The figure shows three views and two pictorial views of one solid part (mm, origin at its lowest corner). Answer the questions. A direction names the side the tool comes from. Coordinates: 2 decimals unless noted, no trailing zeros. Order: outer loops, then holes, each group sorted by start corner. A loop starts at its lowest first (then second) coordinate and runs counter-clockwise, first axis right, second up.
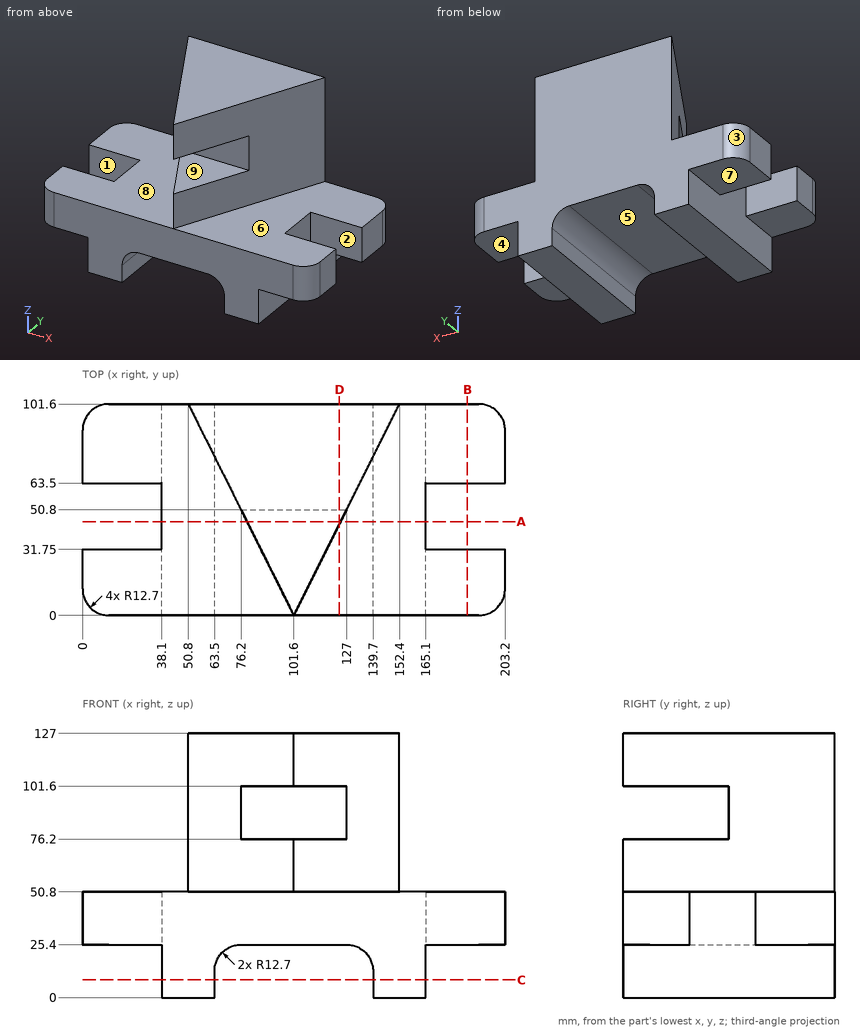
1) Each of these flat-tipped pins is pushed along its axis until it touches: P1, Ø11.5, axis at x = 184, y = 85.5, coming from the -Z side; P2, Ø8, axis at x = 127.5, y = 56.5, coming from the -Z side; P3, Ø14, axis at y = 50, z = 6, coming from the -X side. Where does it stop, or does it pass through?
2) Straight lines are drawn through the part: probe 1 along Y at (x, z) = (188.5, 48.5); probe 2 along X at (y, z) = (25, 11); probe 3 along Z at (x, y) = (165.5, 28.5). For each, find the intervals that lie inside material, in ascending order.
3) The mould has two halves that part along Y. Classify the marked faces 1, 2, 3 and 4: released by +Y, released by -Y, zero draft, split by the parting line, or undercut.
4) A cutting plane is placed at A-A, the plane y = 45. Write down the section's boundary in (x, z).
5) For the marked faces 5, 6, 7, 8 and 9, determine the directions among +Z, -Z, +X, -X, +Y, -Y from which every point of the face is accessible in a straight line to the end or side of a thin tool.
6) A cutting plane is placed at D-D, the plane x = 123.5. Write down the section's boundary in (y, z).
7) A cutting plane is placed at B-B, the plane x = 185. Write down the section's boundary in (y, z).
8) A cutting plane is placed at C-C, the plane z = 8.5. Write down the section's boundary in (x, y), plus the area to 3 significant figures.
Working result:
1. P1: stops at z = 25.4
1. P2: stops at z = 24.58
1. P3: stops at x = 38.1
2. probe 1: y = 0 to 31.75, 63.5 to 101.6
2. probe 2: x = 38.1 to 63.5, 139.7 to 165.1
2. probe 3: z = 25.4 to 50.8
3. face 1: undercut
3. face 2: undercut
3. face 3: released by +Y
3. face 4: zero draft
4. outline: (38.1, 0) - (63.5, 0) - (63.5, 12.7) arc R12.7 cw to (76.2, 25.4) - (127, 25.4) arc R12.7 cw to (139.7, 12.7) - (139.7, 0) - (165.1, 0) - (165.1, 50.8) - (124.1, 50.8) - (124.1, 76.2) - (79.1, 76.2) - (79.1, 50.8) - (38.1, 50.8) - close; (79.1, 101.6) - (124.1, 101.6) - (124.1, 127) - (79.1, 127) - close
5. face 5: -Z, +Y, -Y
5. face 6: +Z, +X, -Y
5. face 7: -Z, -X, +Y, -Y
5. face 8: +Z, -X, -Y
5. face 9: +X, -X, -Y
6. outline: (0, 25.4) - (101.6, 25.4) - (101.6, 127) - (43.8, 127) - (43.8, 101.6) - (50.8, 101.6) - (50.8, 76.2) - (43.8, 76.2) - (43.8, 50.8) - (0, 50.8) - close
7. outline: (0, 25.4) - (31.75, 25.4) - (31.75, 50.8) - (0, 50.8) - close; (63.5, 25.4) - (101.6, 25.4) - (101.6, 50.8) - (63.5, 50.8) - close
8. outline: (38.1, 0) - (63.5, 0) - (63.5, 101.6) - (38.1, 101.6) - close; (139.7, 0) - (165.1, 0) - (165.1, 101.6) - (139.7, 101.6) - close
8. area: 5,160 mm2
